CAD build for the part. Positions are in the model's coordinates, mm. A direction names the side the tool comes from. Give positions to 0.01 mm unless a question says otherwise; leave off trailing zeros. Order: outer loops, then holes, each group sorted by start corner. A loop starts at its lowest first (then second) coordinate and runs counter-clockwise, first axis right, second up. Notation, with made-up numbers: (49, -9) -> (105, -9) arc R22 cw to (105, 2) -> close; hole circle Ø5 at (12, -36.75). An arc over 180 degrees is marked (long way). Use one line per item in the form item = value. Start each with the question number.
1) Cut at A-A, the plane x = 0. Give the cut face in (y, z).
2) Cut at B-B, the plane y = -47.5. Give the cut face in (x, z), and give its area (3 significant figures).
3) Probe line 1 (Z direction, x = 0, y = -4); line 2 (Y direction, x = 4, z = 8.5); line 3 (Z direction, x = -2, y = -53.5). List the from-to ranges inside material, lowest first.
4) Cut at D-D, the plane z = -5.75. Give the cut face in (x, y).
5) Drop flat-ended pins along their axis: P1, Ø2, axis at x = 0, z = -7, coming from the +Y side; P2, Ø1.5, axis at x = 3.5, y = -21.5, coming from the -Z side; P3, Ø1.2, axis at x = 6.5, z = 3.75, coming from the +Y side. Give the stop position or say it passes through.
6) Tool access for faces 1 (the face through (-6, -56, 0.25)), 2 (the face through (0, -55.7, 0)), 3 (the face through (-7.487, -3.042, 3.62)), 4 (the face through (6, -56, -0.25)), 5 (the face through (6, -56, 0.25)): list every direction of +Z, -Z, +X, -X, +Y, -Y with a clear straight run to the whole face (end or side of a thin tool).
7) Cut at C-C, the plane y = -3. Give the cut face in (x, z).
8) Mould opens along X. For faces 6 (the face through (0, 7, -2)), 7 (the face through (0, 0, -4)), 8 (the face through (0.6, -3, -8.3)), 9 (the face through (0, -6, -8)) say: pulls with the +X half, pulls with the -X half, needs draft (parallel to the pull), parting line crosses it, or undercut.
Autodesk Inventor part; units mm, degrees
ref_plane "YZ Plane" through (0, 0, 0) normal (1, 0, 0) x (0, 1, 0)
ref_plane "XZ Plane" through (0, 0, 0) normal (0, 1, 0) x (-1, 0, 0)
ref_plane "XY Plane" through (0, 0, 0) normal (0, 0, 1) x (1, 0, 0)
sketch "Эскиз1" plane through (0, 0, 0) normal (0, 1, 0) x (-1, 0, 0)
  circle A0 centre (0, 0) radius 10
  circle A1 centre (0, 0) radius 3.5
  circle A2 centre (0, 0) radius 2
  dimension "d0" = 20
  dimension "d1" = 7
  dimension "d2" = 4
extrude "Выдавливание1" add sketch "Эскиз1" against normal blind 21.6 contours A0 | A1 | A2
extrude "Выдавливание2" add sketch "Эскиз1" along normal blind 3 contours A1
extrude "Выдавливание3" add sketch "Эскиз1" along normal blind 10.5 contours A2
sketch "Эскиз2" plane through (0, 10.5, 0) normal (0, 1, 0) x (1, 0, 0)
  circle A0 centre (0, 0) radius 2
  circle A1 centre (0, 0) radius 2
  circle A2 centre (0, 0) radius 3.5
  line L0 (-3.1623, -1.5) -> (3.1623, -1.5)
  point P0 (0, 2)
  point P1 (0, 3.5)
  point P2 (1.3229, -1.5)
  point P3 (-1.3229, -1.5)
  dimension "d9" = 1.5
extrude "Выдавливание4" cut sketch "Эскиз2" against normal blind 7 contours L0 A0 picked at (0.3089, -1.5908)
sketch "Эскиз3" plane through (0, -21.6, 0) normal (0, -1, 0) x (1, 0, 0)
  line L0 (6.3804, -7.7) -> (-6.3804, -7.7)
  line L1 (-6.3804, -7.7) -> (-6.3804, 7.7)
  line L2 (-6.3804, 7.7) -> (6.3804, 7.7)
  line L3 (6.3804, 7.7) -> (6.3804, -7.7)
  circle A0 centre (0, 0) radius 10
  arc A1 (6.3804, -7.7) -> (6.3804, 7.7) centre (0, 0) ccw
  arc A2 (-6.3804, 7.7) -> (-6.3804, -7.7) centre (0, 0) ccw
  line L4 (5.3804, 0.25) -> (7.3804, 0.25)
  line L5 (7.3804, 0.25) -> (7.3804, -0.25)
  line L6 (7.3804, -0.25) -> (5.3804, -0.25)
  line L7 (5.3804, -0.25) -> (5.3804, 0.25)
  line L8 (5.3804, 0.25) -> (7.3804, -0.25) construction
  line L9 (0, -7.7) -> (0, 7.7) construction
  line L10 (-5.3804, 0.25) -> (-7.3804, 0.25)
  line L11 (-7.3804, 0.25) -> (-7.3804, -0.25)
  line L12 (-7.3804, -0.25) -> (-5.3804, -0.25)
  line L13 (-5.3804, -0.25) -> (-5.3804, 0.25)
  point P0 (6.3804, 0)
  point P1 (-6.3804, -7.7)
  dimension "d12" = 15.4
  dimension "d13" = 2
  dimension "d14" = 0.5
extrude "Выдавливание5" add sketch "Эскиз3" along normal blind 36 contours L6 L7 L4 L3 | L3 L4 L5 L6 | L12 L11 L10 L1 | L1 L10 L13 L12
extrude "Выдавливание6" add sketch "Эскиз3" along normal blind 32 contours L0 L1 L12 L13 L10 L2 L3 L4 L7 L6 | L3 L6 L5 L4 A0 | A0 L1 L10 L11 L12
sketch "Эскиз4" plane through (0, -53.6, 0) normal (0, -1, 0) x (1, 0, 0)
  circle A0 centre (0, 0) radius 2
  circle A1 centre (0, 0) radius 3.1
  dimension "d19" = 6.2
extrude "Выдавливание7" add sketch "Эскиз4" along normal blind 2.1 contours A0 | A1
sketch "Эскиз5" plane through (0, 0, 0) normal (0, 1, 0) x (1, 0, 0)
  circle A0 centre (0, 0) radius 3.5
  line L0 (0, 0) -> (0, 7.5) construction
  circle A1 centre (0, 7.5) radius 1 construction
  circle A2 centre (-6.4952, -3.75) radius 1 construction
  circle A3 centre (6.4952, -3.75) radius 1 construction
  dimension "d39" = 2
  dimension "d40" = 7.5
  dimension "d43" = 360
hole "Отверстие3" at (0, 0, -7.5) at (6.4952, 0, 3.75) at (-6.4952, 0, 3.75) direction (0, -1, 0) diameter 2 depth 6
properties part number "motor20" material "Сталь"
Result:
q1.outline = (-55.7, -3.1) -> (-53.6, -3.1) -> (-53.6, -7.7) -> (-21.6, -7.7) -> (-21.6, -10) -> (0, -10) -> (0, -8.5) -> (-6, -8.5) -> (-6, -6.5) -> (0, -6.5) -> (0, -3.5) -> (3, -3.5) -> (3, -2) -> (10.5, -2) -> (10.5, 1.5) -> (3.5, 1.5) -> (3.5, 2) -> (3, 2) -> (3, 3.5) -> (0, 3.5) -> (0, 10) -> (-21.6, 10) -> (-21.6, 7.7) -> (-53.6, 7.7) -> (-53.6, 3.1) -> (-55.7, 3.1) -> close
q2.outline = (-6.38, -7.7) -> (6.38, -7.7) arc R10 ccw to (6.38, 7.7) -> (-6.38, 7.7) arc R10 ccw to start
q2.area = 274 mm²
q3.line_1 = -10 to -8.5, -6.5 to 10
q3.line_2 = -21.6 to 0
q3.line_3 = -7.7 to 7.7
q4.outline = (-8.18, -53.6) -> (8.18, -53.6) -> (8.18, 0) -> (-8.18, 0) -> close
q5.P1 = 0
q5.P2 = -9.61
q5.P3 = -6
q6.face_1 = +Z, -X, -Y
q6.face_2 = +Z, -Z, -Y
q6.face_3 = +Y
q6.face_4 = -Z, +X, -Y
q6.face_5 = +Z, +X, -Y
q7.outline = circle Ø20 at (0, 0); hole circle Ø2 at (-6.5, 3.75); hole circle Ø2 at (0, -7.5); hole circle Ø2 at (6.5, 3.75)
q8.face_6 = parting line crosses it
q8.face_7 = needs draft
q8.face_8 = undercut
q8.face_9 = undercut
